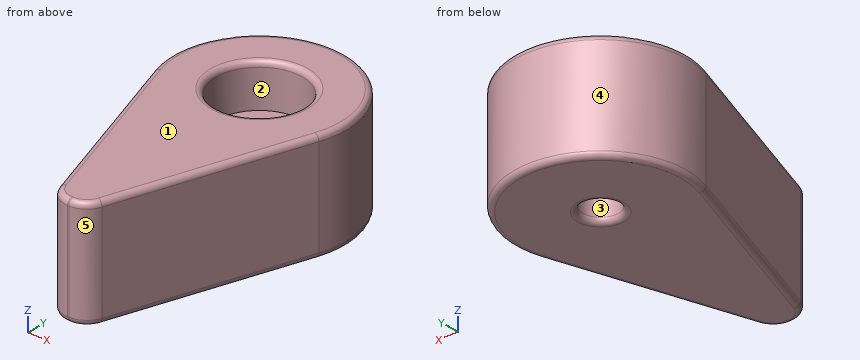
from build123d import *

# Parameters (mm, degrees)
EXTRUDE_1_DEPTH     = 10
FILLET_1_R          = 2
SKETCH_4_R          = 4
CUT_EXTRUDE_1_DEPTH = 4
M4X0_71_D           = 3.3
FILLET_3_R          = 0.5


with BuildPart() as part:
    # Эскиз1 → Бобышка-Вытянуть1 (new body)
    with BuildSketch(Plane.XY):
        with BuildLine():
            Line((-1.5, -21), (-7.597720185, -2.504924749))
            ThreePointArc((-7.597720185, -2.504924749), (0, 8), (7.597720185, -2.504924749))
            Line((7.597720185, -2.504924749), (1.5, -21))
            Line((1.5, -21), (-1.5, -21))
        make_face()
    extrude(amount=EXTRUDE_1_DEPTH)

    # Скругление1
    fillet_1_edges = [part.edges().sort_by_distance(p)[0] for p in [
        (-1.5, -21, 5),
        (1.5, -21, 5),
    ]]
    fillet(fillet_1_edges, radius=FILLET_1_R)

    # Эскиз4 → Вырез-Вытянуть1 (cut)
    with BuildSketch(Plane.XY.offset(10)):
        Circle(SKETCH_4_R)
    extrude(amount=-CUT_EXTRUDE_1_DEPTH, mode=Mode.SUBTRACT)

    # Отверстие обработанное метчиком M4x0.71 (through all)
    with Locations(Plane.XY.offset(6)):
        with Locations((0, 0)):
            Hole(M4X0_71_D / 2)

    # Скругление3
    fillet_3_edges = [part.edges().sort_by_distance(p)[0] for p in [
        (0, 8, 10),
        (-4.77532194, -11.065577968, 10),
        (4.77532194, -11.065577968, 0),
        (4.77532194, -11.065577968, 10),
        (0, -21, 0),
        (-1.225572491, -20.620565083, 0),
        (1.225572491, -20.620565083, 0),
        (0, -21, 10),
        (-1.225572491, -20.620565083, 10),
        (1.225572491, -20.620565083, 10),
        (-4, 0, 10),
        (1.65, 0, 0),
        (-4.77532194, -11.065577968, 0),
        (0, 8, 0),
    ]]
    fillet(fillet_3_edges, radius=FILLET_3_R)


solid = part.part
CAD build for the part. Positions are in the model's coordinates, mm. Face numbers are marked on the shaded views. A direction names the side the tool comes from. Round coordinates to 2 decimals unless told otherwise and drop trailing zeros. Loops run counter-clockwise (first coordinate to the right, second up) from the corner with the lowest first, then second, coordinate; pieces in that order, holes last.
(1) Two-plate mould, pull along X, no slides. Class the marked faces 3, 4 and 5: +X half, -X half, draft (parallel to the pull), parting line (faces both ways), or undercut.
(2) Which spindle directions (+Z, -Z, +X, -X, +Y, -Y) get a long thin tool onto all of the face, cutting with end or side? Do the marked faces 1 and 2. Say none if no direction does.
(3) Drop flat-ended pins along their axis: pin 1 (1 mm diameter, centred on y = 3.5, z = 8.5, fed in from +X); pin 2 (5 mm diameter, centred on y = -4.5, z = 6.5, fed in from +X); pin 3 (3 mm diameter, centred on y = -8.5, z = 6.5, fed in from -X). Give the stop position or say it passes through.
(4) Wall check: line 1 along Y through (x, z) = (0, 4.85); line 2 along Y through (x, z) = (0, 7.6); line 3 along X through (y, z) = (2, 9.25). Give the ranges that are in metal, low to high.
(5) Cut at A-A (z = 5.5). Give the cut face in (x, y).
(6) Cut at B-B (z = 8.5). Give the cut face in (x, y).
Findings below:
1. face 3: undercut
1. face 4: parting line
1. face 5: +X half
2. face 1: +Z, +X, -X, +Y, -Y
2. face 2: +Z
3. pin 1: stops at x = 7.42
3. pin 2: stops at x = 7.75
3. pin 3: stops at x = -6.12
4. line 1: y = -21 to -1.65, 1.65 to 8
4. line 2: y = -21 to -4, 4 to 8
4. line 3: x = -7.75 to -3.46, 3.46 to 7.75
5. outline: (-7.6, -2.5) - (-1.95, -19.63) arc R2 ccw to (-0.05, -21) - (0.05, -21) arc R2 ccw to (1.95, -19.63) - (7.6, -2.5) arc R8 ccw (long way) to start; hole circle Ø3.3 at (0, 0)
6. outline: (-7.6, -2.5) - (-1.95, -19.63) arc R2 ccw to (-0.05, -21) - (0.05, -21) arc R2 ccw to (1.95, -19.63) - (7.6, -2.5) arc R8 ccw (long way) to start; hole circle Ø8 at (0, 0)
